Design review of the part built by this model. Coordinates are the model's own, in mm. A direction names the side the tool comes from. Round coordinates to 2 decimals unless told otherwise and drop trailing zeros. Order: outer loops, then holes, each group sorted by start corner. A loop starts at its lowest first (then second) coordinate and runs counter-clockwise, first axis right, second up. Notation, with made-up numbers: (17.5, 31.5) - (60.5, 31.5) arc R20 ccw to (60.5, 64.5) - close; hole circle Ø10 at (58, 75). An arc over 180 degrees is marked (long way). Answer as a JSON object with one key per item and string values. Group by question number.
from build123d import *

# Parameters (mm, degrees)
F0_W     = 19.5
F0_H     = 26.3
F1_DEPTH = 14.7
F2_R     = 2
F3_R     = 2
F4_DEPTH = 2


with BuildPart() as f1:
    # F0 (on Top) → F1 (new body)
    with BuildSketch(Plane.XY):
        Rectangle(F0_W, F0_H)
        with BuildLine():
            ThreePointArc((-2.949152, -0.55), (0, 3), (2.949152, -0.55))
            Line((2.949152, -0.55), (4.25, -0.55))
            Line((4.25, -0.55), (4.25, -2.45))
            Line((4.25, -2.45), (1.731329, -2.45))
            Line((1.731329, -2.45), (0, -2.45))
            Line((0, -2.45), (-1.731329, -2.45))
            Line((-1.731329, -2.45), (-4.25, -2.45))
            Line((-4.25, -2.45), (-4.25, -0.55))
            Line((-4.25, -0.55), (-2.949152, -0.55))
        make_face(mode=Mode.SUBTRACT)
    extrude(amount=F1_DEPTH)

    # F2
    f2_edges = [f1.edges().sort_by_distance(p)[0] for p in [
        (-9.75, 13.15, 7.35),
        (-9.75, -13.15, 7.35),
        (9.75, -13.15, 7.35),
        (9.75, 13.15, 7.35),
    ]]
    fillet(f2_edges, radius=F2_R)

    # F3
    f3_edges = [f1.edges().sort_by_distance(p)[0] for p in [
        (-9.75, 0, 14.7),
    ]]
    fillet(f3_edges, radius=F3_R)

    # F0 (on Top) → F4 (join)
    with BuildSketch(Plane.XY):
        with BuildLine():
            Line((4.25, -0.55), (2.949152, -0.55))
            ThreePointArc((2.949152, -0.55), (2.525713, -1.61888), (1.731329, -2.45))
            Line((1.731329, -2.45), (4.25, -2.45))
            Line((4.25, -2.45), (4.25, -0.55))
        make_face()
        with BuildLine():
            ThreePointArc((-1.731329, -2.45), (-2.525713, -1.61888), (-2.949152, -0.55))
            Line((-2.949152, -0.55), (-4.25, -0.55))
            Line((-4.25, -0.55), (-4.25, -2.45))
            Line((-4.25, -2.45), (-1.731329, -2.45))
        make_face()
    extrude(amount=F4_DEPTH)


solid = f1.part
1. Take a section at C-C, the plane z = 7.75. Give the boundary of the cut face in (x, y), then the cut area to 3 significant figures.
2. Take a section at B-B, the plane y = 0. Give the boundary of the cut face in (x, z), then the cut area to 3 significant figures.
3. Take a section at A-A, the plane x = 0. Give the boundary of the cut face in (y, z).
4. To check wall thickness, follow line 1 (Y direction, x = -4, z = 4.25); line 2 (X direction, y = -2.25, z = 10); line 3 (X direction, y = 0, z = 6.25). State the ranges of each line that lie inside material, in increasing order. Write a range as from..to.
5. Clearance check with a flat-ended pin moving along its axis: P1, Ø1.5, axis at x = 3, y = -1.5, coming from the +Z side. State where the tip first meets the part, or that it passes through.
6. Tool access review of faces 1 (the flat face through (-3, -2, 2)), 2 (the flat face through (-9.75, 0, 6)): name each direction out of +Z, -Z, +X, -X, +Y, -Y from which nothing blocks a thin tool from reaching the whole face with its end or side.
7. Mouldability with a two-part tool opening along X and no side actions: class faces 3 (the cylindrical face through (9.15, 12.58, 6.44)), 4 (the flat face through (-4.25, -2, 8)), 5 (the cylindrical face through (-0.11, -12.58, 14.1)) as pulls with the +X half, pulls with the -X half, needs draft (parallel to the pull), parting line crosses it, or undercut.
Response values:
{
 "1": {"outline": "(-9.75, -11.15) arc R2 ccw to (-7.75, -13.15) - (7.75, -13.15) arc R2 ccw to (9.75, -11.15) - (9.75, 11.15) arc R2 ccw to (7.75, 13.15) - (-7.75, 13.15) arc R2 ccw to (-9.75, 11.15) - close; hole (-4.25, -2.45) - (4.25, -2.45) - (4.25, -0.55) - (2.95, -0.55) arc R3 ccw (long way) to (-2.95, -0.55) - (-4.25, -0.55) - close", "area": "476 mm2"},
 "2": {"outline": "(-9.75, 0) - (-3, 0) - (-3, 14.7) - (-7.75, 14.7) arc R2 ccw to (-9.75, 12.7) - close; (3, 0) - (9.75, 0) - (9.75, 12.7) arc R2 ccw to (7.75, 14.7) - (3, 14.7) - close", "area": "197 mm2"},
 "3": {"outline": "(-13.15, 0) - (-2.45, 0) - (-2.45, 14.7) - (-11.15, 14.7) arc R2 ccw to (-13.15, 12.7) - close; (3, 0) - (13.15, 0) - (13.15, 12.7) arc R2 ccw to (11.15, 14.7) - (3, 14.7) - close"},
 "4": {"line 1": "-13.15..-2.45, -0.55..13.15", "line 2": "-9.75..-4.25, 4.25..9.75", "line 3": "-9.75..-3, 3..9.75"},
 "5": {"P1": "z = 2"},
 "6": {"face 1": "+Z", "face 2": "+Z, -Z, -X, +Y, -Y"},
 "7": {"face 3": "pulls with the +X half", "face 4": "undercut", "face 5": "needs draft"}
}
